Geometry: see drawing. Coordinates: mm, zero at the bounding-box minimum. A direction names the side the tool comes from. Round coordinates to 2 decimals unless told otherwise and drop trailing zeros. Order: outer loops, then holes, each group sorted by start corner. A loop starts at its lowest first (then second) coordinate and runs counter-clockwise, first axis right, second up. Notation, with made-up numbers: (19, 69) -> (32, 69) arc R11 cw to (32, 81) -> close; hole circle Ø9 at (-5, -32.5). An arc over 180 degrees is marked (long way). One line per item, written item: value. Start each with the question number.
1) Section C-C (z = 37.25). Return the cut outline in (x, y).
2) Section A-A (y = 3.25). Return the cut outline in (x, z), and give its area (3 significant figures).
3) Section D-D (x = 33). Return the cut outline in (y, z).
4) Pin query (flat end, axial travel): P1, Ø5, axis at x = 3.25, z = 3.25, coming from the +Y side; P2, Ø5, axis at x = 37.25, z = 3.25, coming from the -Y side. Return the tip coordinate at first contact, or that it passes through.
5) Section B-B (x = 37.25). Return the cut outline in (y, z), and give its area (3 significant figures).
6) Ray query, L1, parallel to X at y = 4.2, z = 37.25; L2, parallel to Y at x = 29, z = 32.5. Return the intervals inside material, ascending.
7) Reachability of the marked faces 1, 2 and 3 from +Z, -Z, +X, -X, +Y, -Y: full face, straight path, thin tool, end or side. Return the list, or none.
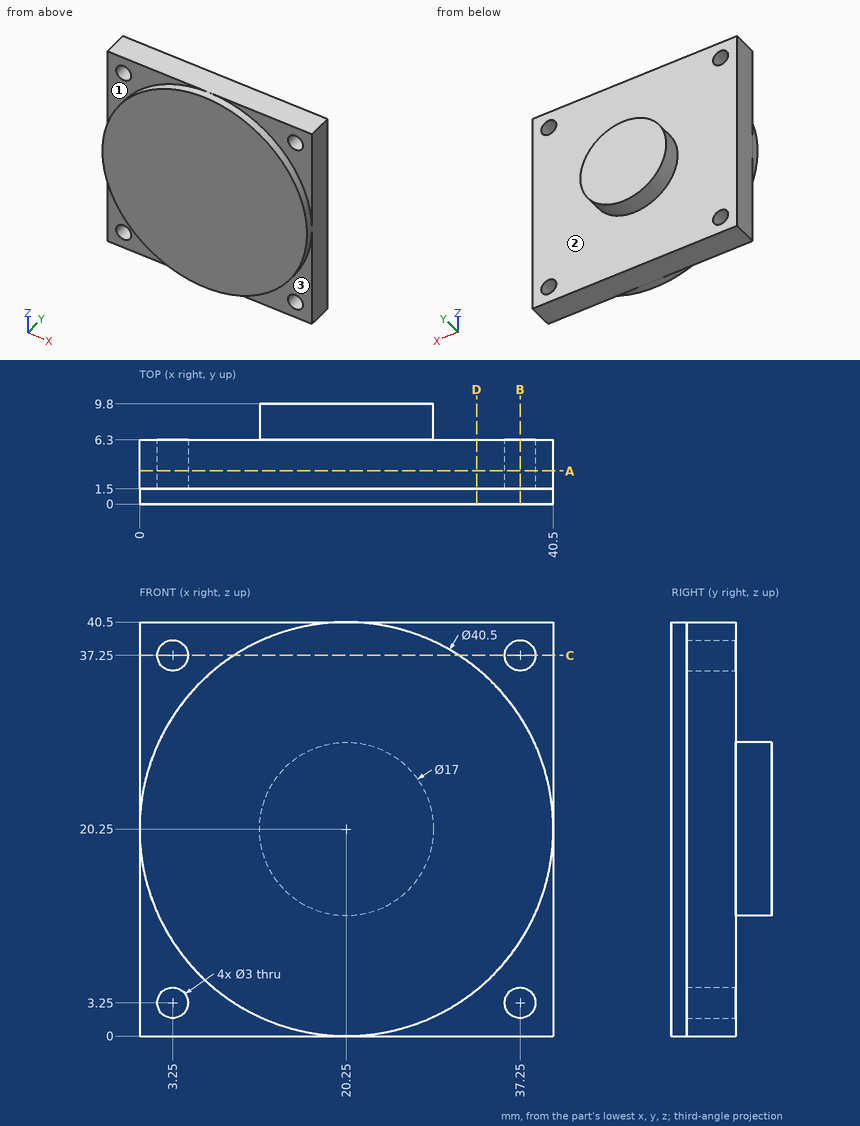
Findings:
1. outline: (0, 1.5) -> (1.75, 1.5) -> (1.75, 6.3) -> (0, 6.3) -> close; (4.75, 1.5) -> (9.25, 1.5) -> (9.25, 0) -> (31.25, 0) -> (31.25, 1.5) -> (35.75, 1.5) -> (35.75, 6.3) -> (4.75, 6.3) -> close; (38.75, 1.5) -> (40.5, 1.5) -> (40.5, 6.3) -> (38.75, 6.3) -> close
2. outline: (0, 0) -> (40.5, 0) -> (40.5, 40.5) -> (0, 40.5) -> close; hole circle Ø3 at (3.25, 3.25); hole circle Ø3 at (3.25, 37.25); hole circle Ø3 at (37.25, 3.25); hole circle Ø3 at (37.25, 37.25)
2. area: 1,610 mm2
3. outline: (0, 4.52) -> (1.5, 4.52) -> (1.5, 0) -> (6.3, 0) -> (6.3, 40.5) -> (1.5, 40.5) -> (1.5, 35.98) -> (0, 35.98) -> close
4. P1: y = 6.3
4. P2: y = 1.5
5. outline: (0, 9.25) -> (1.5, 9.25) -> (1.5, 4.75) -> (6.3, 4.75) -> (6.3, 35.75) -> (1.5, 35.75) -> (1.5, 31.25) -> (0, 31.25) -> close; (1.5, 0) -> (6.3, 0) -> (6.3, 1.75) -> (1.5, 1.75) -> close; (1.5, 38.75) -> (6.3, 38.75) -> (6.3, 40.5) -> (1.5, 40.5) -> close
5. area: 199 mm2
6. L1: 0 to 1.75, 4.75 to 35.75, 38.75 to 40.5
6. L2: 0 to 6.3
7. face 1: +Z, -X, -Y
7. face 2: +Y
7. face 3: -Z, +X, -Y
